Geometry: see drawing. Coordinates: mm, zero at the bounding-box minimum. Round coordinates to 2 decimals unless told otherwise and drop trailing zeros. Write each loop counter-clockwise with the first axis right and the second up, starting at its lowest first coordinate (ties: lowest second). Pieces come first, ordered by that corner, then holes. Notation, with made-up numbers: M 31,19 L 59,19 A21 cw 59,40 Z; hole C -37,29 d4. An arc over 180 degrees is marked long. Use one line per item in the form item = value. Start each with the question number.
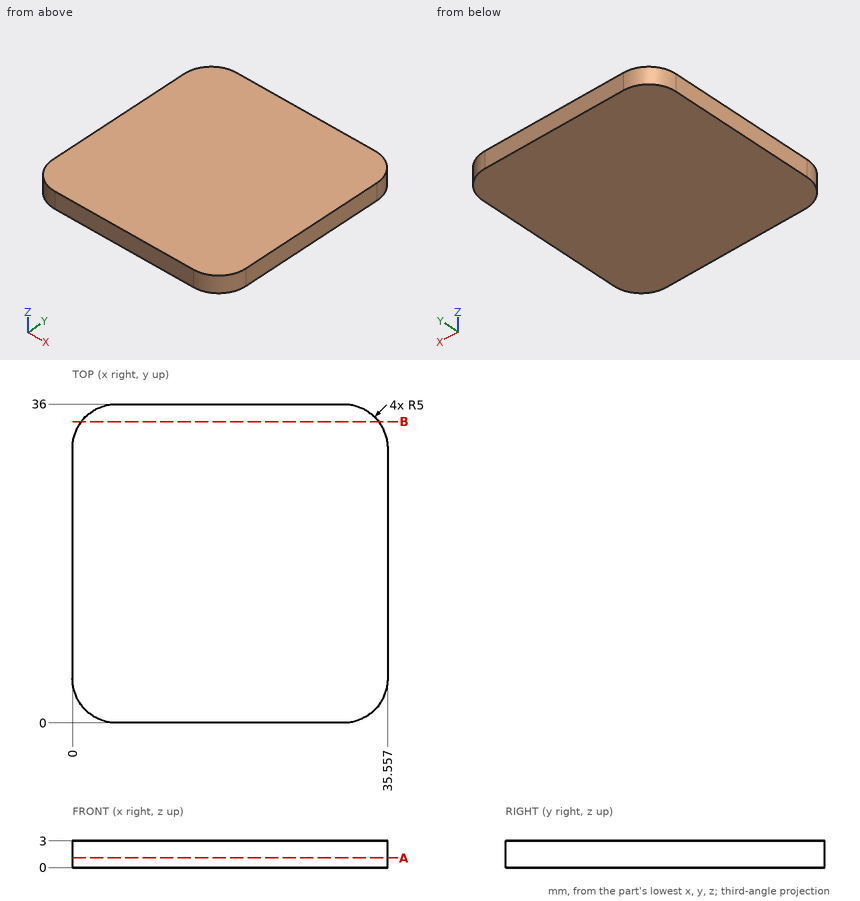
Item 1: Cut plane B-B (y = 34). Output: boundary loops of the cut face in (x, z).
Item 2: Ray query, line 1 (Y direction, x = 34.5, z = 0.7) (1 decimal); line 2 (X direction, y = 2, z = 2.4); line 3 (Y direction, x = 33.5, z = 1.35). Return the intervals inside material, ascending. Write a range as from..to.
Item 3: Cut plane A-A (z = 1.1). Output: boundary loops of the cut face in (x, y).
Final values:
q1.outline = M 1,0 L 34.56,0 L 34.56,3 L 1,3 Z
q2.line_1 = 1.9..34.1
q2.line_2 = 1..34.56
q2.line_3 = 0.96..35.04
q3.outline = M 0,5 A5 ccw 5,0 L 30.56,0 A5 ccw 35.56,5 L 35.56,31 A5 ccw 30.56,36 L 5,36 A5 ccw 0,31 Z
